```python
from build123d import *

# Parameters (mm, degrees)
F0_R     = 1.11278
F1_DEPTH = 5.08


with BuildPart() as f1:
    # F0 (on Top) → F1 (new body)
    with BuildSketch(Plane.XY):
        with BuildLine():
            ThreePointArc((-16.198163, 0), (0, 16.198163), (16.198163, 0))
            Line((16.198163, 0), (29.21493, 0))
            ThreePointArc((29.21493, 0), (28.989076, 3.625685), (28.315007, 7.195311))
            Line((28.315007, 7.195311), (26.650215, 7.298667))
            ThreePointArc((26.650215, 7.298667), (24.176076, 4.107999), (20.300193, 5.239043))
            ThreePointArc((20.300193, 5.239043), (16.461726, 5.366865), (19.487275, 7.732498))
            ThreePointArc((19.487275, 7.732498), (21.951756, 10.930632), (25.83104, 9.811312))
            Line((25.83104, 9.811312), (27.115017, 10.876028))
            ThreePointArc((27.115017, 10.876028), (24.968577, 15.168464), (22.148354, 19.051576))
            Line((22.148354, 19.051576), (20.497724, 18.434355))
            ThreePointArc((20.497724, 18.434355), (19.606952, 14.575136), (15.706482, 13.88711))
            ThreePointArc((15.706482, 13.88711), (12.228664, 12.25771), (13.849808, 15.739384))
            ThreePointArc((13.849808, 15.739384), (14.528579, 19.641475), (18.385674, 20.5414))
            Line((18.385674, 20.5414), (18.998977, 22.19349))
            ThreePointArc((18.998977, 22.19349), (15.233076, 24.92921), (11.080488, 27.032109))
            Line((11.080488, 27.032109), (9.98984, 25.842269))
            ThreePointArc((9.98984, 25.842269), (10.987015, 21.838828), (7.691111, 19.357112))
            ThreePointArc((7.691111, 19.357112), (5.246235, 16.44803), (5.041196, 20.242517))
            ThreePointArc((5.041196, 20.242517), (3.888406, 24.172243), (7.030199, 26.799181))
            Line((7.030199, 26.799181), (6.842575, 28.402312))
            ThreePointArc((6.842575, 28.402312), (0, 29.21493), (-6.842575, 28.402312))
            Line((-6.842575, 28.402312), (-7.030199, 26.799181))
            ThreePointArc((-7.030199, 26.799181), (-3.888406, 24.172243), (-5.041196, 20.242517))
            ThreePointArc((-5.041196, 20.242517), (-5.246235, 16.44803), (-7.691111, 19.357112))
            ThreePointArc((-7.691111, 19.357112), (-10.987015, 21.838828), (-9.98984, 25.842269))
            Line((-9.98984, 25.842269), (-11.080488, 27.032109))
            ThreePointArc((-11.080488, 27.032109), (-15.233076, 24.92921), (-18.998977, 22.19349))
            Line((-18.998977, 22.19349), (-18.385674, 20.5414))
            ThreePointArc((-18.385674, 20.5414), (-14.528579, 19.641475), (-13.849808, 15.739384))
            ThreePointArc((-13.849808, 15.739384), (-12.228664, 12.25771), (-15.706482, 13.88711))
            ThreePointArc((-15.706482, 13.88711), (-19.606952, 14.575136), (-20.497724, 18.434355))
            Line((-20.497724, 18.434355), (-22.148354, 19.051576))
            ThreePointArc((-22.148354, 19.051576), (-24.890954, 15.295507), (-27.002761, 11.151817))
            Line((-27.002761, 11.151817), (-25.705667, 9.954591))
            ThreePointArc((-25.705667, 9.954591), (-21.861689, 10.899789), (-19.487275, 7.732498))
            ThreePointArc((-19.487275, 7.732498), (-16.461726, 5.366865), (-20.300193, 5.239043))
            ThreePointArc((-20.300193, 5.239043), (-24.085137, 4.079831), (-26.633381, 7.109026))
            Line((-26.633381, 7.109026), (-28.38687, 6.906354))
            ThreePointArc((-28.38687, 6.906354), (-29.007176, 3.477909), (-29.21493, 0))
            Line((-29.21493, 0), (-16.198163, 0))
        make_face()
        with Locations((0, 27.872039)):
            Circle(F0_R, mode=Mode.SUBTRACT)
    extrude(amount=F1_DEPTH)


solid = f1.part
```
Geometry: final body of the model. Coordinates: model frame, mm. A direction names the side the tool comes from. Coordinates: 2 decimals unless noted, no trailing zeros. Loops run counter-clockwise (first coordinate to the right, second up) from the corner with the lowest first, then second, coordinate; pieces in that order, holes last. Notation, with made-up numbers: (-21, 16) -> (28, 16) arc R17 ccw to (28, 48) -> close; hole circle Ø5 at (-6.75, 60.25). An arc over 180 degrees is marked (long way). Use a Markdown table: item, result. Add a question column.
(1) Section query C-C, the plane y = 23.5. Return loops of the section in (x, z).
(2) Line query: line 1 along Y through (x, z) = (0, 3.6); line 2 along X through (y, z) = (6.75, 1.35); line 3 along X through (y, z) = (13, 4.75). Output: solid intervals per line, ascending.
(3) Access query for faces 1 (the flat face through (21.335, 18.747, 2.504)), 2 (the flat face through (-27.5, 7.01, 2.5)), 3 (the cylindrical face through (3.87, 24.11, 2.5)), 4 (the flat face through (26.464, 10.336, 2.504)). Directions: +Z, -Z, +X, -X, +Y, -Y. A direction counts if a zero-diameter tool reaches every point of the face in a straight line with its end or side. Return the directions, or none.
(4) Mould query, pull axis Y, two halves, no side actions, for faces 5 (the flat face through (2, 17, 5.08)), 6 (the cylindrical face through (11.01, 21.9, 2.5)), 7 (the cylindrical face through (15.289, 24.895, 2.504)), 8 (the cylindrical face through (-12.18, 12.31, 2.5)). Classes: pulls with the +Y half, pulls with the -Y half, needs draft (parallel to the pull), parting line crosses it, or undercut.
(5) Section query A-A, the plane x = 0. Return loops of the section in (y, z), plus the area to 3 significant figures.
(6) Section query D-D, the plane x = 23. Return loops of the section in (y, z), plus the area to 3 significant figures.
(7) Pin query (flat end, axial travel): pin 1 Ø3 at (y, z) = (7.5, 1.5) entering from +X; pin 2 Ø2 at (x, z) = (-12.5, 0.5) entering from +Y; pin 3 Ø1.5 at (x, z) = (-0.5, 1) entering from -Y. Return the tip coordinate at first contact, or that it passes through.
(8) Section query B-B, the plane y = 17. Return loops of the section in (x, z), plus the area to 3 significant figures.
Answer:
| question | item | result |
|---|---|---|
| 1 | outline | (-17.36, 0) -> (-11.18, 0) -> (-11.18, 5.08) -> (-17.36, 5.08) -> close; (-3.75, 0) -> (3.75, 0) -> (3.75, 5.08) -> (-3.75, 5.08) -> close; (11.18, 0) -> (17.36, 0) -> (17.36, 5.08) -> (11.18, 5.08) -> close |
| 2 | line 1 | y = 16.2 to 26.76, 28.98 to 29.21 |
| 2 | line 2 | x = -28.42 to -26.57, -16.5 to -14.72, 14.72 to 16.5, 26.57 to 28.42 |
| 2 | line 3 | x = -26.16 to -15.59, -11.75 to -9.66, 9.66 to 11.75, 15.59 to 26.16 |
| 3 | face 1 | +Z, -Z, +Y |
| 3 | face 2 | +Z, -Z, -X |
| 3 | face 3 | +Z, -Z |
| 3 | face 4 | +Z, -Z, +X |
| 4 | face 5 | needs draft |
| 4 | face 6 | undercut |
| 4 | face 7 | pulls with the +Y half |
| 4 | face 8 | undercut |
| 5 | outline | (16.2, 0) -> (26.76, 0) -> (26.76, 5.08) -> (16.2, 5.08) -> close; (28.98, 0) -> (29.21, 0) -> (29.21, 5.08) -> (28.98, 5.08) -> close |
| 5 | area | 54.8 mm^2 |
| 6 | outline | (0, 0) -> (3.93, 0) -> (3.93, 5.08) -> (0, 5.08) -> close; (11.11, 0) -> (18.01, 0) -> (18.01, 5.08) -> (11.11, 5.08) -> close |
| 6 | area | 55.1 mm^2 |
| 7 | pin 1 | stops at x = 28.59 |
| 7 | pin 2 | stops at y = 26.86 |
| 7 | pin 3 | stops at y = 16.15 |
| 8 | outline | (-23.76, 0) -> (-20.72, 0) -> (-20.72, 5.08) -> (-23.76, 5.08) -> close; (-13.55, 0) -> (-7.39, 0) -> (-7.39, 5.08) -> (-13.55, 5.08) -> close; (-4.39, 0) -> (4.39, 0) -> (4.39, 5.08) -> (-4.39, 5.08) -> close; (7.39, 0) -> (13.55, 0) -> (13.55, 5.08) -> (7.39, 5.08) -> close; (20.72, 0) -> (23.76, 0) -> (23.76, 5.08) -> (20.72, 5.08) -> close |
| 8 | area | 138 mm^2 |
